Can you work these out from the model? Positions are in its coordinate system, mm. A direction names the side the tool comes from. Give positions to 0.01 mm unless a question says otherwise; leave off trailing zeros. Loops run counter-clockwise (first coordinate to the right, second up) from the corner with the lowest first, then second, coordinate; pieces in that order, holes last. Notation, with made-up numbers: M -31.75,29 L -18.75,29 A14 ccw -18.75,56 Z; hole C 2.25,83.5 d2. An arc over 180 degrees is marked long. Put each result on its own line as item: value. Start each with the question number.
1) Imagine slicing it at C-C (y = -0.5). Write out the boundary of the cut face in (x, z).
2) Imagine slicing it at A-A (x = -3.25). Write out the boundary of the cut face in (y, z), then the cut area to 3 significant figures.
3) Imagine slicing it at B-B (z = 0). Write out the boundary of the cut face in (x, y), then the cut area to 3 significant figures.
4) Imagine slicing it at D-D (x = 0). Write out the boundary of the cut face in (y, z).
5) For P1, Ø2, axis at x = -0.5, y = -8, coming from the -Z side; P2, Ø2, axis at x = -4, z = 3.5, coming from the +Y side; P3, Ø2, axis at x = -4, y = -8, coming from the -Z side, each with a flat end and sliding along its axis, tell me the tip position at first contact or that it passes through.
6) If we mould it in two halves opening along X, with no side actions, what happens to faces 1 (the flat face through (2, -10.922, 2)), 2 (the flat face through (0, -7.366, 0)), 3 (the cylindrical face through (-0.77, -8.6, 3.47))? For each: +X half, -X half, draft (parallel to the pull), parting line (faces both ways), or undercut.
7) For faces 4 (the flat face through (1.54, -9.17, -1.17)), 5 (the flat face through (3, 0, 0)), 6 (the flat face through (1.784, 15.519, 0.746)), which set-ups out of +Z, -Z, +X, -X, +Y, -Y let a thin tool reach every point of the face, with its end or its side?
8) Please list where these lines run through material, in increasing order: line 1 along Y through (x, z) = (-3, 1.5); line 2 along Y through (x, z) = (-4, 4); line 3 along Z through (x, y) = (0.25, 2.5). Write a range as from..to.
from build123d import *

# Parameters (mm, degrees)
SKETCH1_R           = 6.35
BOSS_EXTRUDE1_DEPTH = 6.35
SKETCH2_R           = 2.54
BOSS_EXTRUDE2_DEPTH = 6.35
SKETCH3_R           = 3.556
BOSS_EXTRUDE3_DEPTH = 4.572
CUT_EXTRUDE1_DEPTH  = 3.556


with BuildPart() as part:
    # Sketch1 → Boss-Extrude1 (new body)
    with BuildSketch(Plane(origin=(0, 0, 0), x_dir=(1, 0, 0), z_dir=(0, 1, 0))):
        Circle(SKETCH1_R)
    extrude(amount=BOSS_EXTRUDE1_DEPTH)

    # Sketch2 → Boss-Extrude2 (add)
    with BuildSketch(Plane(origin=(0, 6.35, 0), x_dir=(1, 0, 0), z_dir=(0, 1, 0))):
        Circle(SKETCH2_R)
    boss_extrude2 = extrude(amount=BOSS_EXTRUDE2_DEPTH)

    # Sketch3 → Boss-Extrude3 (add)
    with BuildSketch(Plane(origin=(0, 12.7, 0), x_dir=(1, 0, 0), z_dir=(0, 1, 0))):
        Circle(SKETCH3_R)
    boss_extrude3 = extrude(amount=BOSS_EXTRUDE3_DEPTH)

    # Sketch4 → Cut-Extrude1 (cut)
    with BuildSketch(Plane(origin=(0, 17.272, 0), x_dir=(1, 0, 0), z_dir=(0, 1, 0))):
        Polygon((2.212562326, 0.301992807), (0.84474772, 2.067131585), (-1.367814605, 1.765138778), (-2.212562326, -0.301992807), (-0.84474772, -2.067131585), (1.367814605, -1.765138778), align=None)
    cut_extrude1 = extrude(amount=-CUT_EXTRUDE1_DEPTH, mode=Mode.SUBTRACT)

    # Mirror1: Boss-Extrude2, Boss-Extrude3, Cut-Extrude1 across plane
    add(boss_extrude2.mirror(Plane.ZX.offset(3.175)))
    add(boss_extrude3.mirror(Plane.ZX.offset(3.175)))
    add(cut_extrude1.mirror(Plane.ZX.offset(3.175)), mode=Mode.SUBTRACT)


solid = part.part
Recorded:
1. outline: C 0,0 d5.08
2. outline: M -10.92,-1.44 L -6.35,-1.44 L -6.35,1.44 L -10.92,1.44 Z; M 0,-5.46 L 6.35,-5.46 L 6.35,5.46 L 0,5.46 Z; M 12.7,-1.44 L 17.27,-1.44 L 17.27,1.44 L 12.7,1.44 Z
2. area: 95.7 mm²
3. outline: M -6.35,0 L -2.54,0 L -2.54,-6.35 L -3.56,-6.35 L -3.56,-10.92 L -2.09,-10.92 L -2.09,-7.37 L 2.09,-7.37 L 2.09,-10.92 L 3.56,-10.92 L 3.56,-6.35 L 2.54,-6.35 L 2.54,0 L 6.35,0 L 6.35,6.35 L 2.54,6.35 L 2.54,12.7 L 3.56,12.7 L 3.56,17.27 L 2.09,17.27 L 2.09,13.72 L -2.09,13.72 L -2.09,17.27 L -3.56,17.27 L -3.56,12.7 L -2.54,12.7 L -2.54,6.35 L -6.35,6.35 Z
3. area: 180 mm²
4. outline: M -10.92,-3.56 L -6.35,-3.56 L -6.35,-2.54 L 0,-2.54 L 0,-6.35 L 6.35,-6.35 L 6.35,-2.54 L 12.7,-2.54 L 12.7,-3.56 L 17.27,-3.56 L 17.27,-1.95 L 13.72,-1.95 L 13.72,1.95 L 17.27,1.95 L 17.27,3.56 L 12.7,3.56 L 12.7,2.54 L 6.35,2.54 L 6.35,6.35 L 0,6.35 L 0,2.54 L -6.35,2.54 L -6.35,3.56 L -10.92,3.56 L -10.92,1.95 L -7.37,1.95 L -7.37,-1.95 L -10.92,-1.95 Z
5. P1: z = -3.56
5. P2: y = 6.35
5. P3: z = -1.91
6. face 1: draft
6. face 2: undercut
6. face 3: parting line
7. face 4: -Y
7. face 5: none
7. face 6: +Y
8. line 1: -10.92..-6.35, 0..6.35, 12.7..17.27
8. line 2: 0..6.35
8. line 3: -6.35..6.35
